```python
from build123d import *

# Parameters (mm, degrees)
F0_W     = 40.084
F0_H     = 45.72
F1_DEPTH = 32.615
F2_T     = -1.5
F3_R     = 12.7
F5_DEPTH = 25.4


with BuildPart() as f1:
    # F0 (on Front) → F1 (new body, symmetric)
    with BuildSketch(Plane.XZ):
        with Locations((20.042, -22.86)):
            Rectangle(F0_W, F0_H)
    extrude(amount=F1_DEPTH, both=True)

    # F2
    f2_openings = [f1.faces().sort_by_distance(p)[0] for p in [
        (20.042, 0, 0),
    ]]
    offset(amount=F2_T, openings=f2_openings)

    # F3
    f3_edges = [f1.edges().sort_by_distance(p)[0] for p in [
        (38.584, 31.115, -22.11),
        (38.584, -31.115, -22.11),
        (40.084, -32.615, -22.86),
        (40.084, 32.615, -22.86),
    ]]
    fillet(f3_edges, radius=F3_R)

    # F4 (on face) → F5 (cut)
    with BuildSketch(Plane.XY.offset(-44.22)):
        with BuildLine():
            Line((11.5, -21.115), (25.884, -21.115))
            ThreePointArc((25.884, -21.115), (27.7931883092, -20.3241883092), (28.584, -18.415))
            Line((28.584, -18.415), (28.584, 18.415))
            ThreePointArc((28.584, 18.415), (27.7931883092, 20.3241883092), (25.884, 21.115))
            Line((25.884, 21.115), (11.5, 21.115))
            Line((11.5, 21.115), (11.5, -21.115))
        make_face()
    extrude(amount=-F5_DEPTH, mode=Mode.SUBTRACT)


solid = f1.part
```
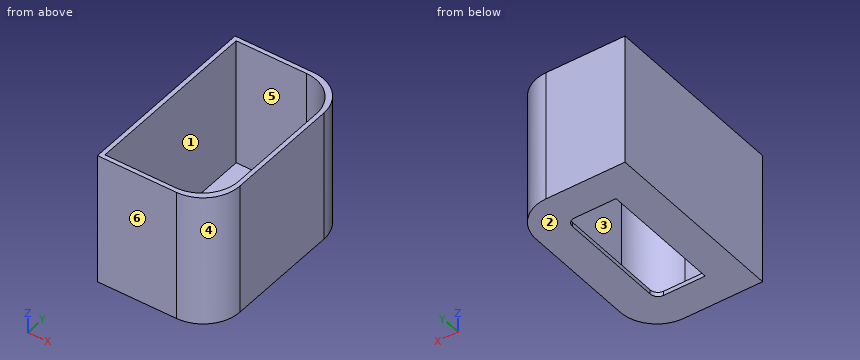
Check sheet for the modelled part. Datum: model origin and axes. Units: mm. Face numbers are marked on the shaded views. A direction names the side the tool comes from. Coordinates: 2 decimals unless noted, no trailing zeros. Write each loop counter-clockwise with the first axis right and the second up, starting at its lowest first coordinate (ties: lowest second). Pieces come first, ordered by that corner, then holes. Notation, with made-up numbers: (-5.5, 57) -> (35.5, 57) arc R30 ccw to (35.5, 88) -> close; hole circle Ø10 at (85, 73). An arc over 180 degrees is marked (long way). Use a Markdown table: item, result.
1. Sectioned sample at B-B (x = 15.5). Enter the section's corners in (y, z) (3 decimals).
Reported:
| item | result |
|---|---|
| outline | (-32.615, -45.72) -> (-21.115, -45.72) -> (-21.115, -44.22) -> (-31.115, -44.22) -> (-31.115, 0) -> (-32.615, 0) -> close; (21.115, -45.72) -> (32.615, -45.72) -> (32.615, 0) -> (31.115, 0) -> (31.115, -44.22) -> (21.115, -44.22) -> close |
2. Sectioned sample at D-D (x = 4). Enter the section's corners in (y, z) (3 decimals).
Reported:
| item | result |
|---|---|
| outline | (-32.615, -45.72) -> (32.615, -45.72) -> (32.615, 0) -> (31.115, 0) -> (31.115, -44.22) -> (-31.115, -44.22) -> (-31.115, 0) -> (-32.615, 0) -> close |
3. Scan lines: line 1 along Y through (x, z) = (19, -33) (3 decimals); line 2 along X through (y, z) = (8.5, -44); line 3 along Z through (x, y) = (31.5, -8). Record each from-to range of solid material in increasing order.
Reported:
| item | result |
|---|---|
| line 1 | y = -32.615 to -31.115, 31.115 to 32.615 |
| line 2 | x = 0 to 1.5, 38.58 to 40.08 |
| line 3 | z = -45.72 to -44.22 |
4. Sectioned sample at A-A (y = 0). Enter the section's corners in (x, z).
Reported:
| item | result |
|---|---|
| outline | (0, -45.72) -> (11.5, -45.72) -> (11.5, -44.22) -> (1.5, -44.22) -> (1.5, 0) -> (0, 0) -> close; (28.58, -45.72) -> (40.08, -45.72) -> (40.08, 0) -> (38.58, 0) -> (38.58, -44.22) -> (28.58, -44.22) -> close |
5. Sectioned sample at C-C (z = -37). Enter the section's corners in (x, y) (3 decimals), plus the area to 3 significant figures.
Reported:
| item | result |
|---|---|
| outline | (0, -32.615) -> (27.384, -32.615) arc R12.7 ccw to (40.084, -19.915) -> (40.084, 19.915) arc R12.7 ccw to (27.384, 32.615) -> (0, 32.615) -> close; hole (1.5, -31.115) -> (25.884, -31.115) arc R12.7 ccw to (38.584, -18.415) -> (38.584, 18.415) arc R12.7 ccw to (25.884, 31.115) -> (1.5, 31.115) -> close |
| area | 307 mm2 |
6. Tool access check on the marked faces 1 and 2. Record the directions out of +Z, -Z, +X, -X, +Y, -Y that give a thin tool (end or side, any length) a straight path to the whole face; none if there is none.
Reported:
| item | result |
|---|---|
| face 1 | +Z |
| face 2 | -Z, +X, -X, +Y, -Y |
7. Release check for a two-part mould opening along X. For the marked faces 3, 4, 5 and 6 record: pulls with the +X half, pulls with the -X half, needs draft (parallel to the pull), parting line crosses it, or undercut.
Reported:
| item | result |
|---|---|
| face 3 | undercut |
| face 4 | pulls with the +X half |
| face 5 | undercut |
| face 6 | needs draft |
8. Go/stop test with flat-tipped pins: pin 1 Ø4 at (x, z) = (34.5, -19.5) entering from -Y; pin 2 Ø1.5 at (x, y) = (6.5, 13.5) entering from +Z; pin 3 Ø10 at (x, y) = (19, -7) entering from +Z; pin 4 Ø4 at (y, z) = (-24, -32.5) entering from +X. Record where each tip stops, or that it passes through.
Reported:
| item | result |
|---|---|
| pin 1 | stops at y = -31.54 |
| pin 2 | stops at z = -44.22 |
| pin 3 | passes through |
| pin 4 | stops at x = 39.91 |
